Could you check a few things on this model? Use its own coordinates, in mm. A direction names the side the tool comes from. Give positions to 0.01 mm unless a question says otherwise; leave off trailing zeros. Loops run counter-clockwise (first coordinate to the right, second up) from the corner with the lowest first, then second, coordinate; pieces in that order, holes last. Notation, with made-up numbers: M 33,16.25 L 83,16.25 A6 cw 83,24.25 Z; hole C 82.5,2.5 d1. An arc over 180 degrees is marked long. Return JSON: item names as keys, results as strings. Group by question number.
1. Please list where these lines run through material, in increasing order: line 1 (Y direction, x = -43, z = -24); line 2 (Y direction, x = -51.5, z = -24); line 3 (Y direction, x = -16, z = -23.75).
2. If we section it at D-D (y = 110.5): Write out the boundary of the cut face in (x, z).
3. If we mould it in two halves opening along Y, with no side actions, what happens to faces 5 (the flat face through (-56, 137, -22.128)), 6 (the flat face through (-13.156, 84, -26)), 7 (the cylindrical face through (-12.119, 170.523, -26.555))? For each: +Y half, -Y half, draft (parallel to the pull), parting line (faces both ways), or undercut.
4. For pin 1 (3 mm diameter, centred on y = 83, z = -25, fed in from +X); pin 2 (2.5 mm diameter, centred on x = -36.9, z = -25.86, fed in from +Y); pin 3 (0.9 mm diameter, centred on x = -55.5, y = 64, fed in from +Z), each with a flat end and sliding along its axis, tell me the tip position at first contact or that it passes through.
5. If we section it at B-B (y = 83): Write out the boundary of the cut face in (x, z), plus the area to 3 significant figures.
6. If we section it at A-A (x = -25): Write out the boundary of the cut face in (y, z), plus the area to 3 significant figures.
7. If we section it at C-C (z = -25.86): State how many separate pieces and enclosed holes the cut face has, plus the area to 3 significant figures.
8. For faces 1 (the flat face through (-13.156, 103, -26)), 2 (the cylindrical face through (-38.403, 60.465, -25.926)), 3 (the flat face through (-37, 86.738, -26)), 4 (the cylindrical face through (-57.526, 62.578, -25.541)), which set-ups out of +Z, -Z, +X, -X, +Y, -Y let a thin tool reach every point of the face, with its end or its side?
```python
from build123d import *

# Parameters (mm, degrees)
BOSS_EXTRUDE1_DEPTH = 2
SKETCH2_R           = 3.556
SKETCH2_R_2         = 1.5
SKETCH2_R_3         = 4.318
SKETCH2_R_4         = 4.064
SKETCH2_R_5         = 3.937
SKETCH2_W           = 47.498
SKETCH2_H           = 5.002835781
SKETCH2_H_2         = 5.760841202
BOSS_EXTRUDE2_DEPTH = 6.732423
BOSS_EXTRUDE3_DEPTH = 6.732423
SKETCH4_R           = 1.5
CUT_EXTRUDE1_DEPTH  = 10
SKETCH5_R           = 1.5
CUT_EXTRUDE2_DEPTH  = 10
SKETCH6_R           = 2.95
SKETCH6_R_2         = 1.5
BOSS_EXTRUDE5_DEPTH = 5
SKETCH7_R           = 2.995
SKETCH7_R_2         = 1.5
BOSS_EXTRUDE6_DEPTH = 5


with BuildPart() as part:
    # Sketch1 → Boss-Extrude1 (new body)
    with BuildSketch(Plane.XY.offset(-28.86000007)):
        with BuildLine():
            Line((-10.615664433, 166.948874967), (-10.615664433, 62.013874967))
            ThreePointArc((-10.615664433, 62.013874967), (-12.080130527, 58.478341061), (-15.615664433, 57.013874967))
            Line((-15.615664433, 57.013874967), (-58.193664433, 57.013874967))
            ThreePointArc((-58.193664433, 57.013874967), (-61.729198339, 58.478341061), (-63.193664433, 62.013874967))
            Line((-63.193664433, 62.013874967), (-63.193664433, 166.948874967))
            ThreePointArc((-63.193664433, 166.948874967), (-61.729198339, 170.484408873), (-58.193664433, 171.948874967))
            Line((-58.193664433, 171.948874967), (-15.615664433, 171.948874967))
            ThreePointArc((-15.615664433, 171.948874967), (-12.080130527, 170.484408873), (-10.615664433, 166.948874967))
        make_face()
    extrude(amount=-BOSS_EXTRUDE1_DEPTH)

    # Sketch2 → Boss-Extrude2 (add)
    with BuildSketch(Plane.XY.offset(-28.86000007)):
        with Locations((-17.219664433, 165.852874967)):
            Circle(SKETCH2_R)
        with Locations((-17.219664433, 165.852874967)):
            Circle(SKETCH2_R_2, mode=Mode.SUBTRACT)
        with Locations((-56.335664433, 136.642874967)):
            Circle(SKETCH2_R_3)
        with Locations((-17.219664433, 63.490874967)):
            Circle(SKETCH2_R_4)
        with Locations((-17.219664433, 63.490874967)):
            Circle(SKETCH2_R_2, mode=Mode.SUBTRACT)
        with Locations((-56.335664433, 63.490874967)):
            Circle(SKETCH2_R_5)
        with Locations((-56.335664433, 63.490874967)):
            Circle(SKETCH2_R_2, mode=Mode.SUBTRACT)
        with Locations((-36.904664433, 102.883892021)):
            Rectangle(SKETCH2_W, SKETCH2_H)
        with Locations((-36.904664433, 83.857955944)):
            Rectangle(SKETCH2_W, SKETCH2_H_2)
    extrude(amount=BOSS_EXTRUDE2_DEPTH)

    # Sketch3 → Boss-Extrude3 (add)
    with BuildSketch(Plane.XY.offset(-28.86000007)):
        with BuildLine():
            Line((-29.404664433, 169.948874967), (-44.404664433, 169.948874967))
            Line((-44.404664433, 169.948874967), (-53.70076371, 167.92637168))
            ThreePointArc((-53.70076371, 167.92637168), (-57.137277803, 169.366456558), (-59.972550774, 166.948874967))
            Line((-59.972550774, 166.948874967), (-61.193664433, 166.948874967))
            Line((-61.193664433, 166.948874967), (-63.193664433, 166.948874967))
            ThreePointArc((-63.193664433, 166.948874967), (-61.729198339, 170.484408873), (-58.193664433, 171.948874967))
            Line((-58.193664433, 171.948874967), (-44.404664433, 171.948874967))
            Line((-44.404664433, 171.948874967), (-29.404664433, 171.948874967))
            Line((-29.404664433, 171.948874967), (-15.615664433, 171.948874967))
            ThreePointArc((-15.615664433, 171.948874967), (-12.080130527, 170.484408873), (-10.615664433, 166.948874967))
            Line((-10.615664433, 166.948874967), (-12.615664433, 166.948874967))
            Line((-12.615664433, 166.948874967), (-13.836778091, 166.948874967))
            ThreePointArc((-13.836778091, 166.948874967), (-16.672051062, 169.366456558), (-20.108565155, 167.92637168))
            Line((-20.108565155, 167.92637168), (-29.404664433, 169.948874967))
        make_face()
        with BuildLine():
            Line((-58.193664433, 57.013874967), (-15.615664433, 57.013874967))
            ThreePointArc((-15.615664433, 57.013874967), (-12.080130527, 58.478341061), (-10.615664433, 62.013874967))
            Line((-10.615664433, 62.013874967), (-12.615664433, 62.013874967))
            Line((-12.615664433, 62.013874967), (-13.433562612, 62.013874967))
            ThreePointArc((-13.433562612, 62.013874967), (-17.971122415, 59.496953723), (-21.283664433, 63.490874967))
            Line((-21.283664433, 63.490874967), (-21.283664433, 59.013874967))
            Line((-21.283664433, 59.013874967), (-52.398664433, 59.013874967))
            Line((-52.398664433, 59.013874967), (-52.398664433, 63.490874967))
            ThreePointArc((-52.398664433, 63.490874967), (-55.583298569, 59.626432626), (-59.985108226, 62.013874967))
            Line((-59.985108226, 62.013874967), (-61.193664433, 62.013874967))
            Line((-61.193664433, 62.013874967), (-63.193664433, 62.013874967))
            ThreePointArc((-63.193664433, 62.013874967), (-61.729198339, 58.478341061), (-58.193664433, 57.013874967))
        make_face()
    extrude(amount=BOSS_EXTRUDE3_DEPTH)

    # Sketch4 → Cut-Extrude1 (cut)
    with BuildSketch(Plane.XZ.offset(-57.013874967)):
        with Locations((-36.904664433, -25.86000007)):
            Circle(SKETCH4_R)
    extrude(amount=-CUT_EXTRUDE1_DEPTH, mode=Mode.SUBTRACT)

    # Sketch5 → Cut-Extrude2 (cut)
    with BuildSketch(Plane(origin=(0, 171.948874967, 0), x_dir=(1, 0, 0), z_dir=(0, 1, 0))):
        with Locations((-36.904664433, 25.86000007)):
            Circle(SKETCH5_R)
    extrude(amount=-CUT_EXTRUDE2_DEPTH, mode=Mode.SUBTRACT)

    # Sketch6 → Boss-Extrude5 (add)
    with BuildSketch(Plane.XZ.offset(-169.948874967)):
        with Locations((-36.904664433, -25.86000007)):
            Circle(SKETCH6_R)
        with Locations((-36.904664433, -25.86000007)):
            Circle(SKETCH6_R_2, mode=Mode.SUBTRACT)
    extrude(amount=BOSS_EXTRUDE5_DEPTH)

    # Sketch7 → Boss-Extrude6 (add)
    with BuildSketch(Plane(origin=(0, 59.013874967, 0), x_dir=(1, 0, 0), z_dir=(0, 1, 0))):
        with Locations((-36.904664433, 25.86000007)):
            Circle(SKETCH7_R)
        with Locations((-36.904664433, 25.86000007)):
            Circle(SKETCH7_R_2, mode=Mode.SUBTRACT)
    extrude(amount=BOSS_EXTRUDE6_DEPTH)


solid = part.part
```
Answer:
{
 "1": {"line 1": "y = 57.01 to 59.01, 80.98 to 86.74, 100.38 to 105.39, 169.95 to 171.95", "line 2": "y = 57.01 to 59.01, 80.98 to 86.74, 100.38 to 105.39, 168.41 to 171.95", "line 3": "y = 57.01 to 62.62, 64.36 to 67.37, 80.98 to 86.74, 100.38 to 105.39, 162.51 to 164.98, 166.73 to 171.95"},
 "2": {"outline": "M -63.19,-30.86 L -10.62,-30.86 L -10.62,-28.86 L -63.19,-28.86 Z"},
 "3": {"face 5": "draft", "face 6": "undercut", "face 7": "+Y half"},
 "4": {"pin 1": "stops at x = -13.16", "pin 2": "stops at y = 105.39", "pin 3": "stops at z = -28.86"},
 "5": {"outline": "M -63.19,-30.86 L -10.62,-30.86 L -10.62,-28.86 L -13.16,-28.86 L -13.16,-22.13 L -60.65,-22.13 L -60.65,-28.86 L -63.19,-28.86 Z", "area": "425 mm²"},
 "6": {"outline": "M 57.01,-30.86 L 171.95,-30.86 L 171.95,-22.13 L 168.99,-22.13 L 168.99,-28.86 L 105.39,-28.86 L 105.39,-22.13 L 100.38,-22.13 L 100.38,-28.86 L 86.74,-28.86 L 86.74,-22.13 L 80.98,-22.13 L 80.98,-28.86 L 59.01,-28.86 L 59.01,-22.13 L 57.01,-22.13 Z", "area": "336 mm²"},
 "7": {"separate pieces": "7", "enclosed holes": "3", "area": "985 mm²"},
 "8": {"face 1": "+Z, +X", "face 2": "-Y", "face 3": "+Z, +X, -X", "face 4": "+Z"}
}
